from build123d import *

# Parameters (mm, degrees)
BOSS_EXTRUDE1_DEPTH = 41.55
SKETCH2_W           = 12.292893219
SKETCH2_H           = 12.292893219
CUT_EXTRUDE1_DEPTH  = 13.25
FILLET1_R           = 4
FILLET2_R           = 1
FILLET3_R           = 0.2
SKETCH3_W           = 13
SKETCH3_H           = 1.8
SKETCH3_W_2         = 1.8
SKETCH3_H_2         = 13
CUT_EXTRUDE2_DEPTH  = 35
SKETCH4_R           = 6.5
CUT_EXTRUDE3_DEPTH  = 35
SKETCH5_R           = 6.5
CUT_EXTRUDE4_DEPTH  = 35
SKETCH6_R           = 2
CUT_EXTRUDE5_DEPTH  = 10.3


with BuildPart() as part:
    # Sketch1 → Boss-Extrude1 (new body)
    with BuildSketch(Plane(origin=(0, 0, 0), x_dir=(1, 0, 0), z_dir=(0, 1, 0))):
        Polygon((0, 0), (0, -40), (13, -40), (13, -13), (35, -13), (35, 0), align=None)
    extrude(amount=BOSS_EXTRUDE1_DEPTH)

    # Sketch2 → Cut-Extrude1 (cut)
    with BuildSketch(Plane(origin=(0, 41.55, 0), x_dir=(1, 0, 0), z_dir=(0, 1, 0))):
        with Locations((6.14644661, -6.14644661)):
            Rectangle(SKETCH2_W, SKETCH2_H)
    extrude(amount=-CUT_EXTRUDE1_DEPTH, mode=Mode.SUBTRACT)

    # Fillet1
    fillet1_edges = [part.edges().sort_by_distance(p)[0] for p in [
        (12.292893219, 28.3, 6.146446609),
    ]]
    fillet(fillet1_edges, radius=FILLET1_R)

    # Fillet2
    fillet2_edges = [part.edges().sort_by_distance(p)[0] for p in [
        (35, 20.775, 0),
        (35, 20.775, 13),
        (13, 20.775, 13),
        (13, 20.775, 40),
        (0, 20.775, 40),
        (6.5, 41.55, 40),
        (0, 41.55, 26.146446609),
        (0, 14.15, 0),
        (0, 28.3, 6.146446609),
        (0, 34.925, 12.292893219),
        (35, 41.55, 6.5),
        (4.146446609, 28.3, 0),
        (12.292893219, 36.925, 0),
        (11.121320344, 29.471572875, 0),
        (23.646446609, 41.55, 0),
        (35, 0, 6.5),
        (24, 0, 13),
        (13, 0, 26.5),
        (6.5, 0, 40),
        (0, 0, 20),
        (17.5, 0, 0),
    ]]
    fillet(fillet2_edges, radius=FILLET2_R)

    # Fillet3
    fillet3_edges = [part.edges().sort_by_distance(p)[0] for p in [
        (12.292893219, 41.55, 6.646446609),
        (6.646446609, 41.55, 12.292893219),
        (13, 41.55, 26.5),
        (24, 41.55, 13),
        (13.292893219, 41.55, 13.292893219),
        (12.646048907, 41.196048907, 39.763296017),
        (0.236703983, 41.196048907, 12.646844311),
        (34.763296017, 41.196048907, 12.646048907),
        (12.646844311, 41.196048907, 0.236703983),
    ]]
    fillet(fillet3_edges, radius=FILLET3_R)

    # Sketch3 → Cut-Extrude2 (cut)
    with BuildSketch(Plane(origin=(0, 41.55, 0), x_dir=(1, 0, 0), z_dir=(0, 1, 0))):
        with Locations((6.5, -30.1)):
            Rectangle(SKETCH3_W, SKETCH3_H)
        with Locations((25.1, -6.5)):
            Rectangle(SKETCH3_W_2, SKETCH3_H_2)
    extrude(amount=-CUT_EXTRUDE2_DEPTH, mode=Mode.SUBTRACT)

    # Sketch4 → Cut-Extrude3 (cut)
    with BuildSketch(Plane.XY.offset(13)):
        with Locations((23, 17)):
            Circle(SKETCH4_R)
    extrude(amount=-CUT_EXTRUDE3_DEPTH, mode=Mode.SUBTRACT)

    # Sketch5 → Cut-Extrude4 (cut)
    with BuildSketch(Plane(origin=(13, 0, 0), x_dir=(0, 0, -1), z_dir=(1, 0, 0))):
        with Locations((-27, 27)):
            Circle(SKETCH5_R)
    extrude(amount=-CUT_EXTRUDE4_DEPTH, mode=Mode.SUBTRACT)

    # Sketch6 → Cut-Extrude5 (cut)
    with BuildSketch(Plane.XZ):
        with Locations(Location((5, 27.5, 0), (0, 0, 270))):
            Circle(SKETCH6_R)
        with Locations(Location((5, 15, 0), (0, 0, 270))):
            Circle(SKETCH6_R)
        with Locations(Location((29, 6, 0), (0, 0, 270))):
            Circle(SKETCH6_R)
    extrude(amount=-CUT_EXTRUDE5_DEPTH, mode=Mode.SUBTRACT)


solid = part.part
Here's how the part is built. I have some questions about the finished solid (model axes, mm). A direction names the side the tool comes from. Coordinates: 2 decimals unless noted, no trailing zeros. Order: outer loops, then holes, each group sorted by start corner. A loop starts at its lowest first (then second) coordinate and runs counter-clockwise, first axis right, second up.
Item 1: For P1, Ø12, axis at x = 31, z = 7, coming from the -Y side; P2, Ø10, axis at x = 23.5, y = 29.5, coming from the +Z side; P3, Ø3, axis at x = 7, y = 39, coming from the -Z side; P4, Ø7, axis at y = 35, z = 7.5, coming from the -X side, each with a flat end and sliding along its axis, tell me the tip position at first contact or that it passes through.
Result sheet:
P1: stops at y = 0
P2: stops at z = 13
P3: stops at z = 12.29
P4: stops at x = 12.21
Item 2: If we section it at C-C on z = 27.5: List the corners of the cut face in (x, y) for me, plus the area to 3 significant figures.
Result sheet:
outline: (0, 1) arc R1 ccw to (1, 0) - (3, 0) - (3, 10.3) - (7, 10.3) - (7, 0) - (12, 0) arc R1 ccw to (13, 1) - (13, 20.52) - (0, 20.52) - close; (0, 33.48) - (13, 33.48) - (13, 41.35) arc R0.2 ccw to (12.8, 41.55) - (1, 41.55) arc R1 ccw to (0, 40.55) - close
area: 330 mm2
Item 3: I need wall thicknesses on line 1 (X direction, y = 6.5, z = 27.5); line 2 (X direction, y = 8.25, z = 6); line 3 (Z direction, x = 3, y = 11). Which ranges of each line are inside material? Lowest first, please.
Result sheet:
line 1: x = 0 to 3, 7 to 13
line 2: x = 0 to 24.2, 26 to 27, 31 to 35
line 3: z = 0 to 29.2, 31 to 40
Item 4: If we mould it in two halves opening along X, with no side actions, what happens to faces 6 (the face through (12.293, 37, 7)), 7 (the face through (13, 21, 24)), 8 (the face through (7, 35, 12.293)), 9 (the face through (26, 32, 7))? For each: +X half, -X half, draft (parallel to the pull), parting line (faces both ways), or undercut.
Result sheet:
face 6: -X half
face 7: +X half
face 8: draft
face 9: undercut
Item 5: If we section it at A-A on y = 6: List the corners of the cut face in (x, z) for me, plus the area to 3 significant figures.
Result sheet:
outline: (0, 1) arc R1 ccw to (1, 0) - (34, 0) arc R1 ccw to (35, 1) - (35, 12) arc R1 ccw to (34, 13) - (14, 13) arc R1 cw to (13, 14) - (13, 39) arc R1 ccw to (12, 40) - (1, 40) arc R1 ccw to (0, 39) - close; hole circle Ø4 at (5, 15); hole circle Ø4 at (5, 27.5); hole circle Ø4 at (29, 6)
area: 767 mm2
Item 6: For faces 1 (the face through (12, 41.55, 15)), 2 (the face through (6, 14, 29.2)), 3 (the face through (26, 9, 7)), 4 (the face through (7, 5, 15)), 5 (the face through (11.09, 29.44, 6.57)), which set-ups out of +Z, -Z, +X, -X, +Y, -Y let a thin tool reach every point of the face, with its end or its side?
Result sheet:
face 1: +Z, -Z, +X, -X, +Y
face 2: +X, -X, +Y
face 3: +Z, -Z, +Y
face 4: -Y
face 5: -Z, -X, +Y
Item 7: If we section it at D-D on z = 36: List the corners of the cut face in (x, y) for me.
Result sheet:
outline: (0, 1) arc R1 ccw to (1, 0) - (12, 0) arc R1 ccw to (13, 1) - (13, 41.35) arc R0.2 ccw to (12.8, 41.55) - (1, 41.55) arc R1 ccw to (0, 40.55) - close
Item 8: If we section it at B-B on x = 23: List the corners of the cut face in (y, z) for me, plus the area to 3 significant figures.
Result sheet:
outline: (0, 1) arc R1 ccw to (1, 0) - (10.5, 0) - (10.5, 13) - (1, 13) arc R1 ccw to (0, 12) - close; (23.5, 0) - (40.55, 0) arc R1 ccw to (41.55, 1) - (41.55, 12.8) arc R0.2 ccw to (41.35, 13) - (23.5, 13) - close
area: 370 mm2
